Solid Edge part; units mm, degrees
sketch "Sketch1" plane through (0, 0, 0) normal (1, 0, 0) x (0, 1, 0)
  arc A0 (2.4972, 42.4266) -> (37.9936, -19.0456) centre (0, 0) cw
  line L0 (81.226, -44.0058) -> (37.9936, -19.0456)
  line L1 (78.726, -48.336) -> (81.226, -44.0058)
  line L2 (35.4939, -23.3759) -> (78.726, -48.336)
  line L3 (-78.7232, -48.3409) -> (-35.4908, -23.3806)
  line L4 (-81.2232, -44.0107) -> (-78.7232, -48.3409)
  line L5 (-37.9911, -19.0507) -> (-81.2232, -44.0107)
  arc A1 (-37.9911, -19.0507) -> (-2.5028, 42.4262) centre (0, 0) cw
  line L6 (-2.5028, 92.3467) -> (-2.5028, 42.4262)
  line L7 (2.4972, 92.3467) -> (-2.5028, 92.3467)
  line L8 (2.4972, 42.4266) -> (2.4972, 92.3467)
  arc A2 (35.4939, -23.3759) -> (-35.4908, -23.3806) centre (0, 0) cw
extrude "Protrusion1" add sketch "Sketch1" along normal mid plane 200
sketch "Sketch2" plane through (0, 0, 0) normal (1, 0, 0) x (0, 1, 0)
  circle A0 centre (0, 0) radius 41
extrude "ExtrudedCutout_5" cut sketch "Sketch2" along normal mid plane 200
sketch "Sketch3" plane through (0, 0, 0) normal (0, -1, 0) x (1, 0, 0)
  circle A0 centre (-75, 0) radius 4
extrude "ExtrudedProtrusion_6" cut sketch "Sketch3" along normal mid plane 90
Design review of the part built by this model. Coordinates are the model's own, in mm. A direction names the side the tool comes from. Coordinates: 2 decimals unless noted, no trailing zeros. Order: outer loops, then holes, each group sorted by start corner. A loop starts at its lowest first (then second) coordinate and runs counter-clockwise, first axis right, second up. Notation, with made-up numbers: (44.5, 68) - (60.5, 68) arc R11 cw to (60.5, 82) - close; hole circle Ø2 at (37, 3). An arc over 180 degrees is marked (long way). One line per question, with ' | ' between items.
Q1. The part is to be moulded in two halves that separate along X. For faces 4 (the cylindrical face through (-71.305, 41.64, -1.532)), 5 (the flat face through (-1, -2.503, 68)), 6 (the flat face through (-100, 18, 38)), say which applies: +X half, -X half, draft (parallel to the pull), parting line (faces both ways), or undercut.
Answer key:
face 4: undercut | face 5: draft | face 6: -X half
Q2. Consider section A-A, the plane z = 0. Give the boundary of the cut face in (x, y), then the cut area to 3 significant figures.
Answer key:
outline: (-100, -42.5) - (-79, -42.5) - (-79, -41) - (-100, -41) - close; (-100, 41) - (-79, 41) - (-79, 42.5) - (-100, 42.5) - close; (-71, -42.5) - (100, -42.5) - (100, -41) - (-71, -41) - close; (-71, 41) - (100, 41) - (100, 42.5) - (-71, 42.5) - close | area: 576 mm2
Q3. To check wall thickness, follow line 1 along Z through (x, y) = (19, 0); line 2 along Y through (x, z) = (-56, 0); line 3 along X through (y, z) = (41.6, 0). State the ranges of each line that lie inside material, in increasing order.
Answer key:
line 1: z = -42.5 to -41, 41 to 92.35 | line 2: y = -42.5 to -41, 41 to 42.5 | line 3: x = -100 to -79, -71 to 100
Q4. Consider section B-B, the plane y = 0. Give the boundary of the cut face in (x, z), then the cut area to 3 significant figures.
Answer key:
outline: (-100, -42.5) - (100, -42.5) - (100, -41) - (-100, -41) - close; (-100, 41) - (100, 41) - (100, 92.35) - (-100, 92.35) - close | area: 10,600 mm2
Q5. For faces 1 (the flat face through (-1, 2.497, 67)), 2 (the flat face through (-1.4, -57.41, -36.035)), 3 (the cylindrical face through (-71.305, -41.64, 1.532)), list the 3-axis set-ups (+Z, -Z, +X, -X, +Y, -Y) from which the entire face can be reached by the end or side of a thin tool; tool diameter is ignored.
Answer key:
face 1: +Z, +X, -X, +Y | face 2: -Z, +X, -X | face 3: +Y, -Y
Q6. Consider section C-C, the plane x = -65.5. Give the boundary of the cut face in (y, z).
Answer key:
outline: (-81.22, -44.01) - (-78.72, -48.34) - (-35.49, -23.38) arc R42.5 ccw to (35.49, -23.38) - (78.73, -48.34) - (81.23, -44.01) - (37.99, -19.05) arc R42.5 ccw to (2.5, 42.43) - (2.5, 92.35) - (-2.5, 92.35) - (-2.5, 42.43) arc R42.5 ccw to (-37.99, -19.05) - close; hole circle Ø82 at (0, 0)
Q7. Clearance check with flat-ended pins moving along their axes: pin 1 Ø25 at (x, z) = (-39, 74.5) entering from +Y; pin 2 Ø10 at (x, z) = (-13, -32) entering from +Y; pin 3 Ø6 at (x, z) = (37, 3) entering from -Y. State where each tip first meets the part, or that it passes through.
Answer key:
pin 1: stops at y = 2.5 | pin 2: stops at y = 69.09 | pin 3: stops at y = -42.5
Q8. Consider section D-D, the plane z = -35. Give the boundary of the cut face in (x, y).
Answer key:
outline: (-100, -65.62) - (100, -65.62) - (100, -55.62) - (-100, -55.62) - close; (-100, -24.11) - (100, -24.11) - (100, -21.35) - (-100, -21.35) - close; (-100, 21.35) - (100, 21.35) - (100, 24.11) - (-100, 24.11) - close; (-100, 55.63) - (100, 55.63) - (100, 65.63) - (-100, 65.63) - close
